from build123d import *

# Parameters (mm, degrees)
F0_R     = 1.016
F1_DEPTH = 3.175


with BuildPart() as f1:
    # F0 (on Front) → F1 (new body)
    with BuildSketch(Plane.XZ):
        with BuildLine():
            Line((11.303, 3.096916), (6.124282, 21.997996))
            ThreePointArc((6.124282, 21.997996), (3.851443, 25.368652), (0, 26.67))
            add(Edge.make_bspline(
                [(0, 26.67), (-11.245353, 29.382879), (-15.981519, -11.110423), (-19.534193, -19.411723)],
                knots=[0, 0, 0, 0, 50.051073, 50.051073, 50.051073, 50.051073], degree=3))
            Line((-19.534193, -19.411723), (-7.62, -19.411723))
            ThreePointArc((-7.62, -19.411723), (-3.445364, -14.272335), (2.54, -11.441027))
            ThreePointArc((2.54, -11.441027), (10.037186, -6.05009), (11.303, 3.096916))
        make_face()
        with BuildLine():
            ThreePointArc((-4.445, 0), (0, 4.445), (4.445, 0))
            ThreePointArc((4.445, 0), (0, -4.445), (-4.445, 0))
        make_face(mode=Mode.SUBTRACT)
        with Locations((-1.950606, 18.954171)):
            Circle(F0_R, mode=Mode.SUBTRACT)
        with Locations((1.950606, 21.685829)):
            Circle(F0_R, mode=Mode.SUBTRACT)
        with BuildLine():
            Line((-7.62, -19.411723), (-19.534193, -19.411723))
            ThreePointArc((-19.534193, -19.411723), (-25.928156, -76.551612), (-2.560215, -129.085307))
            ThreePointArc((-2.560215, -129.085307), (2.045016, -129.592511), (2.624174, -124.995776))
            ThreePointArc((2.624174, -124.995776), (-17.550677, -73.664227), (-7.62, -19.411723))
        make_face()
    extrude(amount=F1_DEPTH)


solid = f1.part
Check sheet for the modelled part. Datum: model origin and axes. Units: mm. Round coordinates to 2 decimals unless told otherwise and drop trailing zeros. Loops run counter-clockwise (first coordinate to the right, second up) from the corner with the lowest first, then second, coordinate; pieces in that order, holes last. Notation, with made-up numbers: (67.25, 51) - (84.25, 51) arc R31 ccw to (84.25, 81) - close; hole circle Ø5 at (16.25, 28.25). An arc over 180 degrees is marked (long way). Answer as CSV lines item,"result". Start each with the question number.
Item 1: Release check for a two-part mould opening along X. For faces 1 (the cylindrical face through (-3.52, -1.57, -14.33)), 2 (the cylindrical face through (-0.96, -1.57, 4.34)), 3 (the cylindrical face through (1.988, -1.565, -129.636)) record: +X half, -X half, draft (parallel to the pull), parting line (faces both ways), or undercut.
Item 2: Depth check by flat-ended pin: P1, Ø14, axis at x = 0, z = 0, coming from the -Y side (3 decimals); P2, Ø1.2, axis at x = -1.95, z = 18.95, coming from the +Y side; P3, Ø1.5, axis at y = -1, z = -70.5, coming from the -X side; P4, Ø1, axis at x = -2, y = -1, coming from the -Z side. Enter the tip coordinate at first touch or a pass-through.
Item 3: Section check C-C (z = -127). Record the boundary of the cut face in (x, y) (3 decimals).
Item 4: Section check A-A (z = -64.5). Record the boundary of the cut face in (x, y) (3 decimals), and give its area (3 significant figures).
Item 5: Scan lines: line 1 (Z direction, x = -4, y = -0.3); line 2 (Z direction, x = 2.5, y = -1.55); line 3 (X direction, y = -1.75, z = 0) (3 decimals). Record each from-to range of solid material in increasing order. Write a range as [from, to].
Item 6: Section check B-B (y = -1.8). Count the separate pieces of the cut face and the enclosed holes in it, and give its area (3 significant figures).
Report:
1,face 1,"+X half"
1,face 2,"undercut"
1,face 3,"parting line"
2,P1,"stops at y = -3.175"
2,P2,"passes through"
2,P3,"stops at x = -26.76"
2,P4,"stops at z = -129.94"
3,outline,"(-4.217, -3.175) - (3.302, -3.175) - (3.302, 0) - (-4.217, 0) - close"
4,outline,"(-27.117, -3.175) - (-18.019, -3.175) - (-18.019, 0) - (-27.117, 0) - close"
4,area,"28.9 mm2"
5,line 1,"z = [-127.28, -115.17], [-14.73, -1.94], [1.94, 25.75]"
5,line 2,"z = [-129.16, -124.83], [-11.45, -3.68], [3.68, 20.83], [22.54, 26.16]"
5,line 3,"x = [-14.646, -4.445], [4.445, 11.72]"
6,separate pieces,"1"
6,enclosed holes,"3"
6,area,"1,840 mm2"
